Design review of the part shown in the three views and the two pictorial views. Dimensions are in mm from the part's minimum x, y and z. Round coordinates to 2 decimals unless told otherwise and drop trailing zeros. Order: outer loops, then holes, each group sorted by start corner. A loop starts at its lowest first (then second) coordinate and runs counter-clockwise, first axis right, second up. Notation, with made-up numbers: M -23,38 L -11,38 A30 ccw -11,62 Z; hole C 68,-23.5 d10. An arc over 180 degrees is marked long. Use a Markdown table: item, result. Add a question column.
(1) Take a section at D-D (z = 10.5). Write out the cut boundary in (x, y), then the cut area to 3 significant figures.
(2) The part is to be moulded in two halves that separate along Z. For the marked faces 1, 2, 3 and 4, say which applies: released by +Z, released by -Z, zero draft, split by the parting line, or undercut.
(3) Take a section at B-B (z = 7.5). Write out the cut boundary in (x, y).
(4) For pin 1 (2.5 mm diameter, centred on y = 3.5, z = 1.5, fed in from +X); pin 2 (0.6 mm diameter, centred on x = 19.5, y = 3, fed in from +Z); pin 3 (2.5 mm diameter, centred on x = 18.5, z = 7.5, fed in from -Y); pin 4 (3.5 mm diameter, centred on x = 3.5, z = 7.5, fed in from +Y), all flat-tipped, find the tip position at first contact; note any pin that passes through.
(5) Take a section at C-C (y = 1.75). Write out the cut boundary in (x, z).
(6) Take a section at A-A (x = 3.5). Count the separate pieces of the cut face and the enclosed holes in it, then the cut area to 3 significant figures.
(7) To check wall thickness, follow probe 1 along X at (y, z) = (1.4, 7.5); probe 2 along X at (y, z) = (1.25, 8); probe 3 along Z at (x, y) = (9, 1.95). State the ranges of each line that lie inside material, in increasing order. Write a range as from..to.
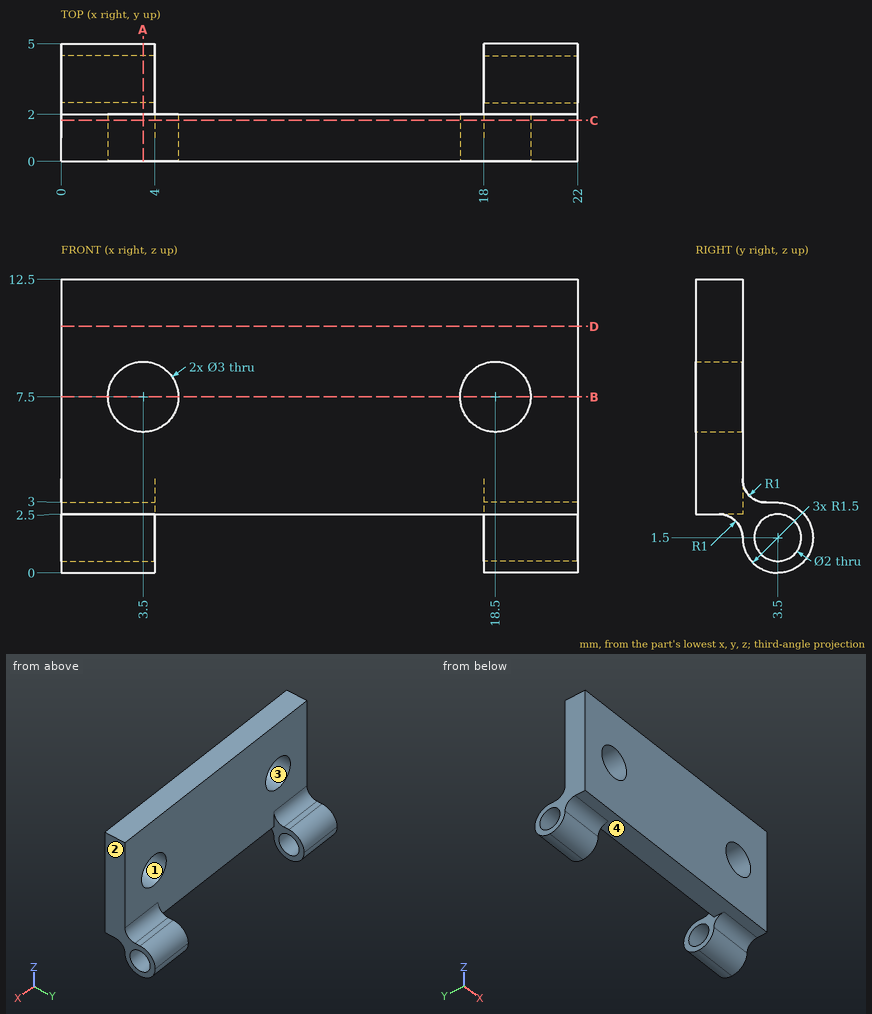
Verdict:
| question | item | result |
|---|---|---|
| 1 | outline | M 0,0 L 22,0 L 22,2 L 0,2 Z |
| 1 | area | 44.0 mm^2 |
| 2 | face 1 | undercut |
| 2 | face 2 | zero draft |
| 2 | face 3 | undercut |
| 2 | face 4 | released by -Z |
| 3 | outline | M 0,0 L 2,0 L 2,2 L 0,2 Z; M 5,0 L 17,0 L 17,2 L 5,2 Z; M 20,0 L 22,0 L 22,2 L 20,2 Z |
| 4 | pin 1 | stops at x = 22 |
| 4 | pin 2 | stops at z = 3.05 |
| 4 | pin 3 | passes through |
| 4 | pin 4 | stops at y = 2 |
| 5 | outline | M 0,2.16 L 4,2.16 L 4,2.5 L 18,2.5 L 18,2.16 L 22,2.16 L 22,12.5 L 0,12.5 Z; hole C 3.5,7.5 d3; hole C 18.5,7.5 d3 |
| 6 | separate pieces | 2 |
| 6 | enclosed holes | 1 |
| 6 | area | 18.8 mm^2 |
| 7 | probe 1 | x = 0..2, 5..17, 20..22 |
| 7 | probe 2 | x = 0..2.09, 4.91..17.09, 19.91..22 |
| 7 | probe 3 | z = 2.5..12.5 |
